from build123d import *

# Parameters (mm, degrees)
F0_W     = 12.7
F0_H     = 50.8
F1_DEPTH = 50.8
F2_W     = 12.7
F2_H     = 12.7
F2_W_2   = 15.875
F2_H_2   = 25.4
F3_DEPTH = 50.801


with BuildPart() as f1:
    # F0 (on Front) → F1 (new body)
    with BuildSketch(Plane.XZ):
        with Locations((6.35, 25.4)):
            Rectangle(F0_W, F0_H)
        Polygon((12.7, 50.8), (12.7, 0), (50.8, 0), (50.8, 25.4), align=None)
    extrude(amount=F1_DEPTH)

    # F2 (on face) → F3 (cut, through all)
    with BuildSketch(Plane(origin=(0, 0, 0), x_dir=(1, 0, 0), z_dir=(0, 0, -1))):
        with Locations((6.35, 44.45)):
            Rectangle(F2_W, F2_H)
        with Locations((6.35, 6.35)):
            Rectangle(F2_W, F2_H)
        with Locations((42.8625, 25.4)):
            Rectangle(F2_W_2, F2_H_2)
    extrude(amount=-F3_DEPTH, mode=Mode.SUBTRACT)


solid = f1.part
Could you check a few things on this model? Use its own coordinates, in mm. A direction names the side the tool comes from. Give positions to 0.01 mm unless a question says otherwise; leave off trailing zeros. Order: outer loops, then holes, each group sorted by start corner. A loop starts at its lowest first (then second) coordinate and runs counter-clockwise, first axis right, second up. Notation, with made-up numbers: M 66.25,73.25 L 125.25,73.25 A19 cw 125.25,104.25 Z; hole C 11.5,-6.75 d9. An arc over 180 degrees is marked long. One line per question, with ' | ' between items.
1. We'd pull the mould along Y, two halves only. Please class faces 4 (the face through (34.925, -25, 18)), 5 (the face through (50.8, -44, 13)), 6 (the face through (31, 0, 20)), 7 (the face through (43, -38.1, 14)): +Y half, -Y half, draft (parallel to the pull), parting line (faces both ways), or undercut.
Results:
face 4: undercut | face 5: draft | face 6: +Y half | face 7: undercut
2. For faces 1 (the face through (6, -12.7, 25)), 2 (the face through (43, -12.7, 14)), 3 (the face through (12.7, -44, 25)), which set-ups out of +Z, -Z, +X, -X, +Y, -Y let a thin tool reach every point of the face, with its end or its side?
Results:
face 1: +Z, -Z, -X, +Y | face 2: +Z, -Z, +X | face 3: +Z, -Z, -X, -Y
3. I'm going to push flat-ended pins straight in: pin 1 (5 mm diameter, centred on x = 9.5, z = 23.5, fed in from +Y); pin 2 (2 mm diameter, centred on y = -14, z = 33, fed in from +X) (3 decimals); pin 3 (10 mm diameter, centred on y = -43.5, z = 15.5, fed in from -X). Where does each tip first touch, or does it pass through?
Results:
pin 1: y = -12.7 | pin 2: x = 34.925 | pin 3: x = 12.7
4. I want a section at D-D (x = 18). List the corners of the cut face in (y, z) for me.
Results:
outline: M -50.8,0 L 0,0 L 0,47.27 L -50.8,47.27 Z
5. I want a section at A-A (z = 28.5). List the corners of the cut face in (x, y) for me (3 decimals).
Results:
outline: M 0,-38.1 L 12.7,-38.1 L 12.7,-50.8 L 46.15,-50.8 L 46.15,-38.1 L 34.925,-38.1 L 34.925,-12.7 L 46.15,-12.7 L 46.15,0 L 12.7,0 L 12.7,-12.7 L 0,-12.7 Z
6. I want a section at B-B (y = -31). List the corners of the cut face in (x, z) for me (3 decimals).
Results:
outline: M 0,0 L 34.925,0 L 34.925,35.983 L 12.7,50.8 L 0,50.8 Z
7. I want a section at C-C (z = 41.5). List the corners of the cut face in (x, y) for me.
Results:
outline: M 0,-38.1 L 12.7,-38.1 L 12.7,-50.8 L 26.65,-50.8 L 26.65,0 L 12.7,0 L 12.7,-12.7 L 0,-12.7 Z
8. If I drill on line 1 (Y direction, x = 36, z = 20.5); line 2 (X direction, y = -35, z = 16.5) (3 decimals); line 3 (Y direction, x = 2, z = 4), over which ranges is the centre line in solid material (lowest first)?
Results:
line 1: -50.8 to -38.1, -12.7 to 0 | line 2: 0 to 34.925 | line 3: -38.1 to -12.7
